```python
from build123d import *

# Parameters (mm, degrees)
SKETCH3_W           = 20
SKETCH3_H           = 17.866253804
BOSS_EXTRUDE1_DEPTH = 30


with BuildPart() as part:
    # Sketch1 → Loft1 section 0
    with BuildSketch(Plane.XY):
        with BuildLine():
            Line((-15, 14.870689655), (15, 14.870689655))
            Line((15, 14.870689655), (15, -14.870689655))
            Line((15, -14.870689655), (-15, -14.870689655))
            Line((-15, -14.870689655), (-15, 14.870689655))
        make_face()
    # Sketch2 → Loft1 section 1
    with BuildSketch(Plane.XY.offset(20)):
        with BuildLine():
            Line((-10, 8.933126902), (10, 8.933126902))
            Line((10, 8.933126902), (10, -8.933126902))
            Line((10, -8.933126902), (-10, -8.933126902))
            Line((-10, -8.933126902), (-10, 8.933126902))
        make_face()
    loft()

    # Sketch3 → Boss-Extrude1 (add)
    with BuildSketch(Plane.XY.offset(20)):
        Rectangle(SKETCH3_W, SKETCH3_H)
    extrude(amount=BOSS_EXTRUDE1_DEPTH)


solid = part.part
```
Read the model definition and answer for the solid it produces. Units are mm, in the model's axes. A direction names the side the tool comes from. Coordinates: 2 decimals unless noted, no trailing zeros. Write each loop counter-clockwise with the first axis right and the second up, starting at its lowest first coordinate (ties: lowest second). Pieces come first, ordered by that corner, then holes. Notation, with made-up numbers: (-29.5, -16) - (13.5, -16) arc R19 cw to (13.5, -10) - close; hole circle Ø2 at (-24, 9.25). An arc over 180 degrees is marked (long way). Answer as a JSON object with one key per item and string values. Group by question number.
1. Consider L1, parallel to X at y = -5.5, z = 47.5; L2, parallel to Y at x = -3, z = 25.5; L3, parallel to X at y = 4, z = 3. Determine where each line is inside the solid, lowest interval first. Write a range as [from, to].
2. A cutting plane is placed at A-A (z = 42). Determine the outline of the cut face in (x, y).
3. Each of these flat-tipped pins is pushed along its axis until it touches: P1, Ø14.5, axis at y = 3.5, z = 33, coming from the +X side; P2, Ø6, axis at x = 5, z = 15.5, coming from the -Y side; P3, Ø10, axis at y = -11, z = 38.5, coming from the -X side; P4, Ø6, axis at y = 12, z = 44.5, coming from the -X side. Where does it stop, or does it pass through?
4. Which of the six approach directions +Z, -Z, +X, -X, +Y, -Y give full straight-line access (tool end or side, diameter ignored) to faces 1 (the flat face through (0, -8.933, 35)), 2 (the flat face through (0, 8.933, 35)), 3 (the flat face through (-10, 0, 35)), 4 (the flat face through (10, 0, 35)), 5 (the flat face through (0, 0, 0))?
Worked out:
{
 "1": {"L1": "x = [-10, 10]", "L2": "y = [-8.93, 8.93]", "L3": "x = [-14.25, 14.25]"},
 "2": {"outline": "(-10, -8.93) - (10, -8.93) - (10, 8.93) - (-10, 8.93) - close"},
 "3": {"P1": "stops at x = 10", "P2": "stops at y = -11.16", "P3": "stops at x = -10", "P4": "passes through"},
 "4": {"face 1": "+Z, +X, -X, -Y", "face 2": "+Z, +X, -X, +Y", "face 3": "+Z, -X, +Y, -Y", "face 4": "+Z, +X, +Y, -Y", "face 5": "-Z, +X, -X, +Y, -Y"}
}
